from build123d import *

# Parameters (mm, degrees)
SKETCH1_W           = 92.7
SKETCH1_H           = 158
SKETCH1_R           = 1.5
BOSS_EXTRUDE1_DEPTH = 3


with BuildPart() as part:
    # Sketch1 → Boss-Extrude1 (new body)
    with BuildSketch(Plane(origin=(0, 3, 0), x_dir=(1, 0, 0), z_dir=(0, 1, 0))):
        Rectangle(SKETCH1_W, SKETCH1_H)
        with Locations((28, -75)):
            Circle(SKETCH1_R, mode=Mode.SUBTRACT)
        with Locations((28, 75)):
            Circle(SKETCH1_R, mode=Mode.SUBTRACT)
        with Locations((-28, 75)):
            Circle(SKETCH1_R, mode=Mode.SUBTRACT)
        with Locations((-28, -75)):
            Circle(SKETCH1_R, mode=Mode.SUBTRACT)
    extrude(amount=-BOSS_EXTRUDE1_DEPTH)


solid = part.part
The model under review builds one solid part; all positions refer to its coordinate system, in mm. Coordinates: 2 decimals unless noted, no trailing zeros. Write each loop counter-clockwise with the first axis right and the second up, starting at its lowest first coordinate (ties: lowest second). Pieces come first, ordered by that corner, then holes. Notation, with made-up numbers: (21, 35) -> (73, 35) arc R20 cw to (73, 39) -> close; hole circle Ø3 at (-5, 6). An arc over 180 degrees is marked (long way). Answer in a Markdown table with one row per item.
1. We need section B-B, the plane z = 75. State the section outline as (x, y) points, and give its area (3 significant figures).
Answers below:
| item | result |
|---|---|
| outline | (-46.35, 0) -> (-29.5, 0) -> (-29.5, 3) -> (-46.35, 3) -> close; (-26.5, 0) -> (26.5, 0) -> (26.5, 3) -> (-26.5, 3) -> close; (29.5, 0) -> (46.35, 0) -> (46.35, 3) -> (29.5, 3) -> close |
| area | 260 mm^2 |
2. Draft analysis for pull direction X (two halves, no side actions). For faces 1 (the cylindrical face through (-29.5, 1.52, -75.07)), 2 (the cylindrical face through (27.805, 1.521, 73.513)), 3 (the flat face through (-46.35, 2, 1)), 4 (the flat face through (-1, 2, 79)), state which applies: +X half, -X half, draft (parallel to the pull), parting line (faces both ways), or undercut.
Answers below:
| item | result |
|---|---|
| face 1 | undercut |
| face 2 | undercut |
| face 3 | -X half |
| face 4 | draft |
3. Clearance check with a flat-ended pin moving along its axis: pin 1 Ø2.5 at (x, z) = (28, 75) entering from -Y. State where the tip first meets the part, or that it passes through.
Answers below:
| item | result |
|---|---|
| pin 1 | passes through |
4. Wall thickness on probe 1 along X at (y, z) = (2.1, 75); probe 2 along Z at (x, y) = (28, 1): over which ranges is each line inside the solid? List them lowest first. Write a range as [from, to].
Answers below:
| item | result |
|---|---|
| probe 1 | x = [-46.35, -29.5], [-26.5, 26.5], [29.5, 46.35] |
| probe 2 | z = [-79, -76.5], [-73.5, 73.5], [76.5, 79] |
5. We need section A-A, the plane x = 28. State the section outline as (y, z) points.
Answers below:
| item | result |
|---|---|
| outline | (0, -79) -> (3, -79) -> (3, -76.5) -> (0, -76.5) -> close; (0, -73.5) -> (3, -73.5) -> (3, 73.5) -> (0, 73.5) -> close; (0, 76.5) -> (3, 76.5) -> (3, 79) -> (0, 79) -> close |
